Answer from the drawing. Dimensions are ordinates in mm from the lowest x, y and z of the part. A direction names the side the tool comes from. Give positions to 0.01 mm unless a question says otherwise; leave off trailing zeros. Write each loop counter-clockwise with the first axis right and the second up, starting at its lowest first coordinate (ties: lowest second). Pieces come first, ordered by that corner, then holes. Notation, with made-up numbers: (61, 2.25) -> (100, 2.25) arc R25 ccw to (100, 22.25) -> close; hole circle Ø11 at (-27, 56). An arc over 180 degrees is marked (long way). Write item = value, one per line.
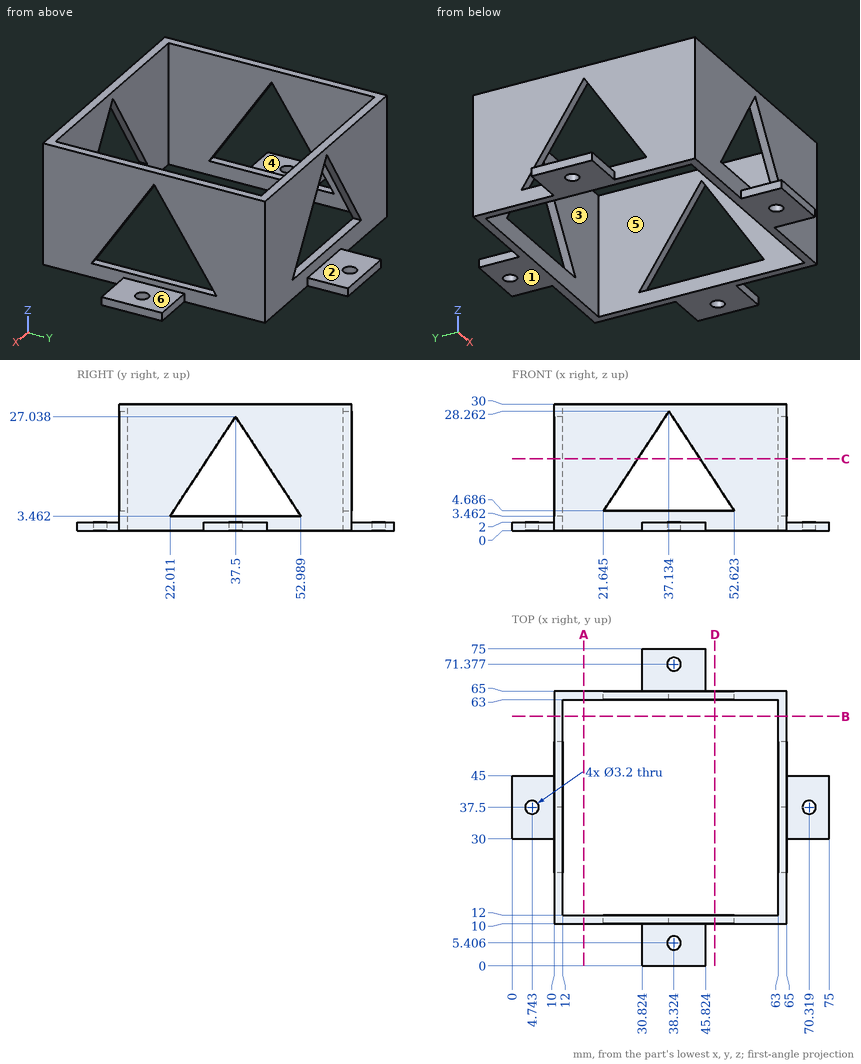
(1) The part is cut by section A-A on x = 17. Determine the outline of the cut face in (y, z), plus the area to 3 significant figures.
Checks:
outline = (10, 0) -> (12, 0) -> (12, 30) -> (10, 30) -> close; (63, 0) -> (65, 0) -> (65, 30) -> (63, 30) -> close
area = 120 mm²
(2) Given P1, Ø12, axis at x = 64.5, z = 7.5, coming from the -Y side; P2, Ø1, axis at x = 5.5, z = 0.5, coming from the -Y side; P3, Ø15, axis at x = 40, z = 16, coming from the +Y side; P4, Ø1.9, axis at x = 38.32, y = 71.38, coming from the -Z side, each flat-ended and moving along its own axis, determine where each tip first touches the part or whether it passes through.
Checks:
P1 = 10
P2 = 30
P3 = 65
P4 = through
(3) For a pull along Y with two mould halves and no side action, classify the marked faces 5 and 6 as released by +Y, released by -Y, zero draft, split by the parting line, or undercut.
Checks:
face_5 = undercut
face_6 = zero draft
(4) Consider L1, parallel to Y at x = 28, z = 24.5; L2, parallel to Z at x = 41.5, y = 64 (1 decimal). Determine where each line is inside the solid, lowest interval first.
Checks:
L1 = 10 to 12, 63 to 65
L2 = 0 to 4.7, 21.6 to 30
(5) A tool of negligible diameter and unlimited length cuts with its end or side. For the marked faces 1, 2, 3 and 4, from which of +Z, -Z, +X, -X, +Y, -Y can it reach the whole face along a straight path? Write none if from no direction.
Checks:
face_1 = -Z, +X, -X, +Y, -Y
face_2 = +Z, +X, -X, +Y
face_3 = +Z, -Z
face_4 = +Z, -X, +Y, -Y
(6) The part is cut by section C-C on z = 17. Determine the outline of the cut face in (x, y) (1 decimal), plus the area to 3 significant figures.
Checks:
outline = (10, 10) -> (29.7, 10) -> (29.7, 12) -> (12, 12) -> (12, 30.9) -> (10, 30.9) -> close; (10, 44.1) -> (12, 44.1) -> (12, 63) -> (29.7, 63) -> (29.7, 65) -> (10, 65) -> close; (44.5, 10) -> (65, 10) -> (65, 30.9) -> (63, 30.9) -> (63, 12) -> (44.5, 12) -> close; (44.5, 63) -> (63, 63) -> (63, 44.1) -> (65, 44.1) -> (65, 65) -> (44.5, 65) -> close
area = 312 mm²
(7) The part is cut by section D-D on x = 48. Determine the outline of the cut face in (y, z).
Checks:
outline = (10, 0) -> (12, 0) -> (12, 4.69) -> (10, 4.69) -> close; (10, 11.72) -> (12, 11.72) -> (12, 30) -> (10, 30) -> close; (63, 0) -> (65, 0) -> (65, 4.69) -> (63, 4.69) -> close; (63, 11.72) -> (65, 11.72) -> (65, 30) -> (63, 30) -> close
